Part model, mm, in its own coordinate system. Face numbers are marked on the shaded views. A direction names the side the tool comes from. Round coordinates to 2 decimals unless told otherwise and drop trailing zeros. Write each loop counter-clockwise with the first axis right and the second up, starting at its lowest first coordinate (ties: lowest second). Pieces come first, ordered by that corner, then holes. Notation, with made-up numbers: (63.25, -24.75) -> (77.25, -24.75) arc R31 ccw to (77.25, 9.25) -> close; hole circle Ø3 at (-11, 53.5). An arc over 180 degrees is marked (long way). Return JSON: item names as keys, results as strings. Group by question number.
(1) Saw through at C-C (z = 0). List the corners of the cut face in (x, y).
(2) Saw through at A-A (x = 0). List the corners of the cut face in (y, z), plus the area to 3 significant figures.
(3) Saw through at B-B (y = 14). List the corners of the cut face in (x, z).
(4) Drill centre lines: L1, parallel to X at y = -39, z = 0; L2, parallel to X at y = -32, z = -7.5; L3, parallel to Y at x = 11.5, z = -10.5. Where is each one in solid material? Low to high. Write a range as from..to.
(5) Mould opens along X. For the marked faces 1, 2, 3 and 4 say: +X half, -X half, draft (parallel to the pull), parting line (faces both ways), or undercut.
(6) Tool access for the marked faces 5, 6, 7 and 8: list every direction of +Z, -Z, +X, -X, +Y, -Y with a clear straight run to the whole face (end or side of a thin tool).
(7) Drop flat-ended pins along their axis: pin 1 Ø10 at (x, y) = (1, 9.5) entering from +Z; pin 2 Ø6 at (x, z) = (20, 13.5) entering from +Y; pin 3 Ø2.5 at (y, z) = (8, -1) entering from -X; pin 4 Ø12 at (x, z) = (-4, 26) entering from -Y. Give the stop position or say it passes through.
(8) Saw through at D-D (y = -85.5). List the corners of the cut face in (x, z), plus the area to 3 significant figures.
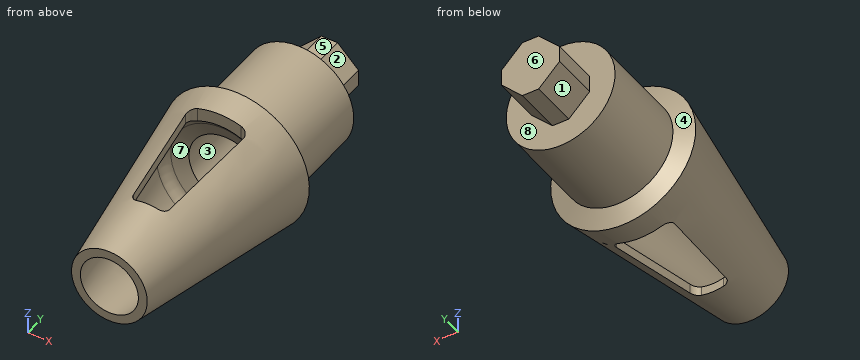
from build123d import *

# Parameters (mm, degrees)
BOSS_EXTRUDE1_DEPTH     = 26
CUT_EXTRUDE1_DEPTH      = 174.481987538
CUT_EXTRUDE1_DEPTH_BACK = 174.481987538


with BuildPart() as part:
    # Sketch1 → Revolve1 (revolve)
    with BuildSketch(Plane.XY, mode=Mode.PRIVATE) as revolve1_sk:
        with BuildLine():
            ThreePointArc((31.66780037, -73.791452413), (30.995225405, -69.840051309), (27.984645692, -67.193858277))
            Line((27.984645692, -67.193858277), (20, -64))
            Line((20, -64), (20, -8))
            Line((20, -8), (0, -8))
            Line((0, -8), (0, 0))
            Line((0, 0), (30, 0))
            Line((30, 0), (30, -50))
            Line((30, -50), (40, -54))
            Line((40, -54), (20.894736842, -164))
            Line((20.894736842, -164), (16, -164))
            Line((16, -164), (31.66780037, -73.791452413))
        make_face()
    revolve(revolve1_sk.sketch.rotate(Axis((0, 95.722418972, 0), (0, -1, 0)), 90), axis=Axis((0, 95.722418972, 0), (0, -1, 0)))

    # Sketch2 → Boss-Extrude1 (add)
    with BuildSketch(Plane(origin=(0, 0, 0), x_dir=(1, 0, 0), z_dir=(0, 1, 0))):
        Polygon((4.506096654, 16), (16, 4.506096654), (16, -4.506096654), (4.506096654, -16), (-4.506096654, -16), (-16, -4.506096654), (-16, 4.506096654), (-4.506096654, 16), align=None)
    extrude(amount=BOSS_EXTRUDE1_DEPTH)

    # Sketch3 → Cut-Extrude1 (cut, two sides: drawn at the far end of the back side and taken through both)
    with BuildSketch(Plane.XY.offset(-CUT_EXTRUDE1_DEPTH_BACK)):
        with BuildLine():
            Line((-12.024465061, -69), (12.024465061, -69))
            ThreePointArc((12.024465061, -69), (15.004977133, -70.332314151), (16, -73.441726104))
            Line((16, -73.441726104), (10, -127.441726104))
            ThreePointArc((10, -127.441726104), (8.692150911, -129.980512072), (6.024465061, -131))
            Line((6.024465061, -131), (-6.024465061, -131))
            ThreePointArc((-6.024465061, -131), (-8.692150911, -129.980512072), (-10, -127.441726104))
            Line((-10, -127.441726104), (-16, -73.441726104))
            ThreePointArc((-16, -73.441726104), (-15.004977133, -70.332314151), (-12.024465061, -69))
        make_face()
    extrude(amount=CUT_EXTRUDE1_DEPTH + CUT_EXTRUDE1_DEPTH_BACK, mode=Mode.SUBTRACT)


solid = part.part
Computed values:
{
 "1": {"outline": "(-40, -54) -> (-20.89, -164) -> (-16, -164) -> (-31.67, -73.79) arc R6 cw to (-27.98, -67.19) -> (-20, -64) -> (-20, -8) -> (20, -8) -> (20, -64) -> (27.98, -67.19) arc R6 cw to (31.67, -73.79) -> (16, -164) -> (20.89, -164) -> (40, -54) -> (30, -50) -> (30, 0) -> (16, 0) -> (16, 26) -> (-16, 26) -> (-16, 0) -> (-30, 0) -> (-30, -50) -> close"},
 "2": {"outline": "(-164, -20.89) -> (-131, -26.63) -> (-131, -21.73) -> (-164, -16) -> close; (-164, 16) -> (-131, 21.73) -> (-131, 26.63) -> (-164, 20.89) -> close; (-69, -37.39) -> (-54, -40) -> (-50, -30) -> (0, -30) -> (0, -16) -> (26, -16) -> (26, 16) -> (0, 16) -> (0, 30) -> (-50, 30) -> (-54, 40) -> (-69, 37.39) -> (-69, 30.43) arc R6 cw to (-67.19, 27.98) -> (-64, 20) -> (-8, 20) -> (-8, -20) -> (-64, -20) -> (-67.19, -27.98) arc R6 cw to (-69, -30.43) -> close", "area": "3,100 mm2"},
 "3": {"outline": "(-16, -4.51) -> (-4.51, -16) -> (4.51, -16) -> (16, -4.51) -> (16, 4.51) -> (4.51, 16) -> (-4.51, 16) -> (-16, 4.51) -> close"},
 "4": {"L1": "-30..-20, 20..30", "L2": "-29.05..-18.54, 18.54..29.05", "L3": "-8..0"},
 "5": {"face 1": "-X half", "face 2": "+X half", "face 3": "undercut", "face 4": "parting line"},
 "6": {"face 5": "+Z, +X, -X, +Y", "face 6": "+Z, -Z, +X, -X, +Y", "face 7": "none", "face 8": "+Y"},
 "7": {"pin 1": "z = 16", "pin 2": "y = 0", "pin 3": "x = -16", "pin 4": "y = -164"},
 "8": {"outline": "(-14.66, -31.26) -> (-14.66, -25.75) arc R29.63 cw to (-14.66, 25.75) -> (-14.66, 31.26) arc R34.53 ccw to start; (14.66, -31.26) arc R34.53 ccw to (14.66, 31.26) -> (14.66, 25.75) arc R29.63 cw to (14.66, -25.75) -> close", "area": "688 mm2"}
}
